Work out the finished part from the listing and answer in its coordinate system (mm). Face numbers are marked on the shaded views. Round coordinates to 2 decimals unless told otherwise and drop trailing zeros. Write each loop counter-clockwise with the first axis right and the second up, starting at its lowest first coordinate (ties: lowest second). Pieces come first, ordered by that corner, then holes. Notation, with made-up numbers: M 14.5,-36 L 38.5,-36 A31 ccw 38.5,-9 Z; hole C 29,83.5 d10. An arc over 180 degrees is marked long. Answer in a Markdown table with one row per item.
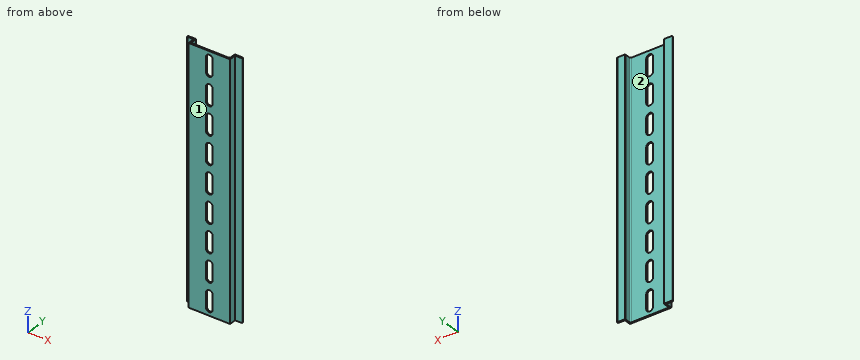
```python
from build123d import *

# Parameters (mm, degrees)
EXTRUDE_THIN1_DEPTH = 90
FILLET1_R           = 1
FILLET2_R           = 0.25
FILLET3_RADIUS      = 0.5
FILLET3_LENGTH      = 180
FILLET4_RADIUS      = 0.5
FILLET4_LENGTH      = 180
CUT_EXTRUDE1_DEPTH  = 93.330926563
LPATTERN1_COUNT     = 5
LPATTERN1_PITCH     = 20
LPATTERN1_COL_COUNT = 5
LPATTERN1_COL_PITCH = 20


with BuildPart() as part:
    # Sketch1 → Extrude-Thin1 (new, symmetric)
    with BuildSketch(Plane.XY):
        Polygon((-20, 5), (-15, 5), (-15, 0), (15, 0), (15, 5), (20, 5), (20, 6), (14, 6), (14, 1), (-14, 1), (-14, 6), (-20, 6), align=None)
    extrude(amount=EXTRUDE_THIN1_DEPTH, both=True)

    # Fillet1
    fillet1_edges = [part.edges().sort_by_distance(p)[0] for p in [
        (-14, 1, 0),
        (14, 1, 0),
    ]]
    fillet(fillet1_edges, radius=FILLET1_R)

    # Fillet2
    fillet2_edges = [part.edges().sort_by_distance(p)[0] for p in [
        (-14, 6, 0),
        (14, 6, 0),
    ]]
    fillet(fillet2_edges, radius=FILLET2_R)

    # Fillet3: full round fillet: the end face becomes a half cylinder, R = half its width
    fillet3_face = Plane((20, 5.5, 0), x_dir=(0, 0, 1), z_dir=(1, 0, 0))  # on the end face: x along it, z out of the body
    fillet3_slab = fillet3_face.offset(-FILLET3_RADIUS / 2) * Box(FILLET3_LENGTH, 2 * FILLET3_RADIUS, FILLET3_RADIUS, mode=Mode.PRIVATE)  # the body's end, R deep
    fillet3_round = Plane((19.5, 5.5, 0), x_dir=(1, 0, 0), z_dir=(0, 0, 1)) * Cylinder(FILLET3_RADIUS, FILLET3_LENGTH, mode=Mode.PRIVATE)  # its axis R under the face
    add(fillet3_slab - fillet3_round, mode=Mode.SUBTRACT)

    # Fillet4: full round fillet: the end face becomes a half cylinder, R = half its width
    fillet4_face = Plane((-20, 5.5, 0), x_dir=(0, 0, 1), z_dir=(-1, 0, 0))  # on the end face: x along it, z out of the body
    fillet4_slab = fillet4_face.offset(-FILLET4_RADIUS / 2) * Box(FILLET4_LENGTH, 2 * FILLET4_RADIUS, FILLET4_RADIUS, mode=Mode.PRIVATE)  # the body's end, R deep
    fillet4_round = Plane((-19.5, 5.5, 0), x_dir=(-1, 0, 0), z_dir=(0, 0, 1)) * Cylinder(FILLET4_RADIUS, FILLET4_LENGTH, mode=Mode.PRIVATE)  # its axis R under the face
    add(fillet4_slab - fillet4_round, mode=Mode.SUBTRACT)

    # Sketch2 → Cut-Extrude1 (cut, through all)
    with BuildSketch(Plane(origin=(0, 1, 0), x_dir=(1, 0, 0), z_dir=(0, 1, 0))):
        with BuildLine():
            Line((-2.5, -5), (-2.5, 5))
            ThreePointArc((-2.5, 5), (0, 7.5), (2.5, 5))
            Line((2.5, 5), (2.5, -5))
            ThreePointArc((2.5, -5), (0, -7.5), (-2.5, -5))
        make_face()
    cut_extrude1 = extrude(amount=-CUT_EXTRUDE1_DEPTH, mode=Mode.SUBTRACT)

    # LPattern1: Cut-Extrude1 ×5
    with Locations(*[(0, 0, -i * LPATTERN1_PITCH) for i in range(1, LPATTERN1_COUNT)]):
        add(cut_extrude1, mode=Mode.SUBTRACT)

    # LPattern1 col: Cut-Extrude1 ×5
    with Locations(*[(0, 0, i * LPATTERN1_COL_PITCH) for i in range(1, LPATTERN1_COL_COUNT)]):
        add(cut_extrude1, mode=Mode.SUBTRACT)


solid = part.part
```
1. The part is cut by section A-A (z = -77.5). Determine the outline of the cut face in (x, y).
Calculated:
| item | result |
|---|---|
| outline | M -19.5,5 L -15,5 L -15,0 L -2.5,0 L -2.5,1 L -13,1 A1 cw -14,2 L -14,5.75 A0.25 ccw -14.25,6 L -19.5,6 A0.5 ccw Z; M 2.5,0 L 15,0 L 15,5 L 19.5,5 A0.5 ccw 19.5,6 L 14.25,6 A0.25 ccw 14,5.75 L 14,2 A1 cw 13,1 L 2.5,1 Z |
2. Consider line 1 along X through (y, z) = (2.1, -16); line 2 along X through (y, z) = (0.5, 21); line 3 along Y through (x, z) = (9.5, 57.5). Determine where each line is inside the solid, lowest interval first. Write a range as from..to.
Calculated:
| item | result |
|---|---|
| line 1 | x = -15..-14, 14..15 |
| line 2 | x = -15..-2.5, 2.5..15 |
| line 3 | y = 0..1 |
3. The part is cut by section C-C (x = 8). Determine the outline of the cut face in (y, z).
Calculated:
| item | result |
|---|---|
| outline | M 0,-90 L 1,-90 L 1,90 L 0,90 Z |
4. The part is cut by section B-B (y = 3.1). Determine the outline of the cut face in (x, z), plus the area to 3 significant figures.
Calculated:
| item | result |
|---|---|
| outline | M -15,-90 L -14,-90 L -14,90 L -15,90 Z; M 14,-90 L 15,-90 L 15,90 L 14,90 Z |
| area | 360 mm² |
5. Given pin 1 (1.1 mm diameter, centred on y = 0.5, z = -1, fed in from -X); pin 2 (1.1 mm diameter, centred on y = 0.5, z = 41, fed in from +X); pin 3 (1.5 mm diameter, centred on y = 4.5, z = 32.5, fed in from -X); pin 4 (1.5 mm diameter, centred on x = -9.5, y = 2, fed in from -Z), each flat-ended and moving along its own axis, determine where each tip first touches the part or whether it passes through.
Calculated:
| item | result |
|---|---|
| pin 1 | stops at x = -15 |
| pin 2 | stops at x = 15 |
| pin 3 | stops at x = -19.93 |
| pin 4 | passes through |
6. Determine the mould class of the marked faces 1 and 2 for opening direction X: released by +X, released by -X, zero draft, split by the parting line, or undercut.
Calculated:
| item | result |
|---|---|
| face 1 | zero draft |
| face 2 | undercut |
7. The part is cut by section D-D (x = 1). Count the separate pieces of the cut face and the enclosed holes in it, plus the area to 3 significant figures.
Calculated:
| item | result |
|---|---|
| separate pieces | 10 |
| enclosed holes | 0 |
| area | 48.8 mm² |
